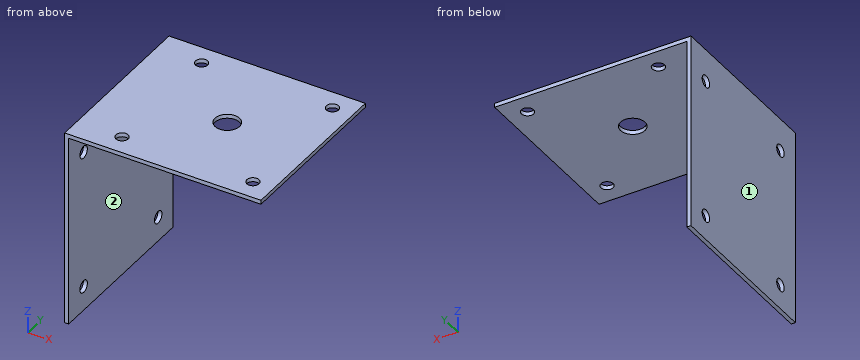
```python
from build123d import *

# Parameters (mm, degrees)
BOSS_EXTRUDE1_DEPTH = 42
SKETCH2_R           = 1.5
SKETCH2_R_2         = 3
CUT_EXTRUDE1_DEPTH  = 42
SKETCH3_R           = 1.5
CUT_EXTRUDE2_DEPTH  = 42


with BuildPart() as part:
    # Sketch1 → Boss-Extrude1 (new body)
    with BuildSketch(Plane(origin=(0, 0, 0), x_dir=(1, 0, 0), z_dir=(0, 1, 0))):
        Polygon((0, 0), (0, 48), (1, 48), (1, 1), (48, 1), (48, 0), align=None)
    extrude(amount=BOSS_EXTRUDE1_DEPTH)

    # Sketch2 → Cut-Extrude1 (cut)
    with BuildSketch(Plane.XY):
        with Locations((11, 37)):
            Circle(SKETCH2_R)
        with Locations((43, 37)):
            Circle(SKETCH2_R)
        with Locations((43, 5)):
            Circle(SKETCH2_R)
        with Locations((11, 5)):
            Circle(SKETCH2_R)
        with Locations((27, 21)):
            Circle(SKETCH2_R_2)
    extrude(amount=-CUT_EXTRUDE1_DEPTH, mode=Mode.SUBTRACT)

    # Sketch3 → Cut-Extrude2 (cut)
    with BuildSketch(Plane(origin=(0, 0, 0), x_dir=(0, 0, -1), z_dir=(1, 0, 0))):
        with Locations((42, 36)):
            Circle(SKETCH3_R)
        with Locations((42, 6)):
            Circle(SKETCH3_R)
        with Locations((8, 6)):
            Circle(SKETCH3_R)
        with Locations((8, 36)):
            Circle(SKETCH3_R)
    extrude(amount=CUT_EXTRUDE2_DEPTH, mode=Mode.SUBTRACT)


solid = part.part
```
CAD build for the part. Positions are in the model's coordinates, mm. Face numbers are marked on the shaded views. A direction names the side the tool comes from. Round coordinates to 2 decimals unless told otherwise and drop trailing zeros. Order: outer loops, then holes, each group sorted by start corner. A loop starts at its lowest first (then second) coordinate and runs counter-clockwise, first axis right, second up. Notation, with made-up numbers: (44, 74.5) - (51, 74.5) arc R23 cw to (51, 109.5) - close; hole circle Ø1 at (20.25, 12.25). An arc over 180 degrees is marked (long way). Use CSV: the item, a comma, the result in double quotes. Start each with the question number.
1) Saw through at D-D (x = 36). List the corners of the cut face in (y, z), and give its area (3 significant figures).
2) Pin check, flat tips, straight feed: pin 1 Ø1 at (y, z) = (28.5, -11) entering from +X; pin 2 Ø4 at (y, z) = (30, -6) entering from -X; pin 3 Ø2.5 at (y, z) = (36, -42) entering from +X; pin 4 Ø21 at (x, y) = (13, 30) entering from -Z. Stop position of each tip, or through.
3) Saw through at C-C (y = 26.5). List the corners of the cut face in (x, z).
4) Tool access for the marked faces 1 and 2: list every direction of +Z, -Z, +X, -X, +Y, -Y with a clear straight run to the whole face (end or side of a thin tool).
5) Saw through at A-A (x = 43). List the corners of the cut face in (y, z).
6) Wall check: L1, parallel to Y at x = 0.75, z = -42; L2, parallel to X at y = 17, z = -23; L3, parallel to Z at x = 15.5, y = 27. Give the ranges that are in metal, low to high. Write a range as [from, to].
7) Saw through at B-B (x = 27). List the corners of the cut face in (y, z), and give its area (3 significant figures).
Values follow:
1,outline,"(0, -1) - (42, -1) - (42, 0) - (0, 0) - close"
1,area,"42.0 mm2"
2,pin 1,"stops at x = 1"
2,pin 2,"stops at x = 0"
2,pin 3,"passes through"
2,pin 4,"stops at z = -1"
3,outline,"(0, -48) - (1, -48) - (1, -1) - (48, -1) - (48, 0) - (0, 0) - close"
4,face 1,"+Z, -Z, -X, +Y, -Y"
4,face 2,"-Z, +X, +Y, -Y"
5,outline,"(0, -1) - (3.5, -1) - (3.5, 0) - (0, 0) - close; (6.5, -1) - (35.5, -1) - (35.5, 0) - (6.5, 0) - close; (38.5, -1) - (42, -1) - (42, 0) - (38.5, 0) - close"
6,L1,"y = [0, 4.5], [7.5, 34.5], [37.5, 42]"
6,L2,"x = [0, 1]"
6,L3,"z = [-1, 0]"
7,outline,"(0, -1) - (18, -1) - (18, 0) - (0, 0) - close; (24, -1) - (42, -1) - (42, 0) - (24, 0) - close"
7,area,"36.0 mm2"
